Model file for the job. Use its own axes, mm. Coordinates: 2 decimals unless noted, no trailing zeros. Order: outer loops, then holes, each group sorted by start corner. A loop starts at its lowest first (then second) coordinate and runs counter-clockwise, first axis right, second up. Notation, with made-up numbers: M 35.5,-3 L 68.5,-3 A19 ccw 68.5,29 Z; hole C 54,61.5 d3. An arc over 180 degrees is marked long. Return JSON: item names as keys, results as strings.
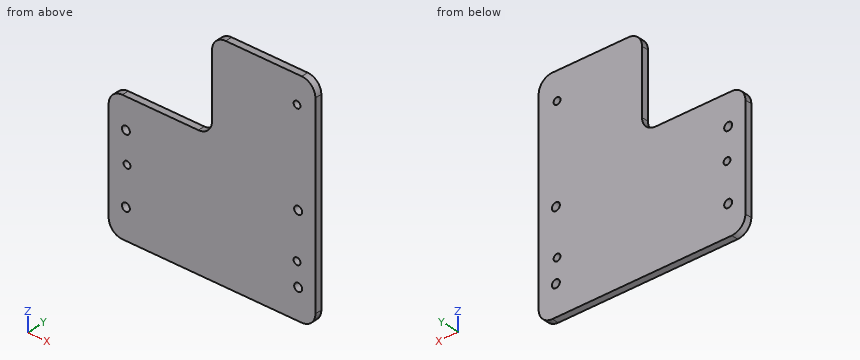
```python
from build123d import *

# Parameters (mm, degrees)
F0_R     = 1.85
F0_R_2   = 1.5875
F1_DEPTH = 3.175


with BuildPart() as f1:
    # F0 (on Front) → F1 (new body)
    with BuildSketch(Plane.XZ):
        with BuildLine():
            ThreePointArc((-48, -23.65), (-46.140128, -28.140128), (-41.65, -30))
            Line((-41.65, -30), (41.65, -30))
            ThreePointArc((41.65, -30), (46.140128, -28.140128), (48, -23.65))
            Line((48, -23.65), (48, 30))
            Line((48, 30), (48, 65.99177))
            ThreePointArc((48, 65.99177), (46.140128, 70.481898), (41.65, 72.34177))
            Line((41.65, 72.34177), (6.35, 72.34177))
            ThreePointArc((6.35, 72.34177), (1.859872, 70.481898), (0, 65.99177))
            Line((0, 65.99177), (0, 36.35))
            ThreePointArc((0, 36.35), (-1.859872, 31.859872), (-6.35, 30))
            Line((-6.35, 30), (-41.65, 30))
            ThreePointArc((-41.65, 30), (-46.140128, 28.140128), (-48, 23.65))
            Line((-48, 23.65), (-48, -23.65))
        make_face()
        with Locations((-40, -16)):
            Circle(F0_R, mode=Mode.SUBTRACT)
        with Locations((-39.4716, 1.8262)):
            Circle(F0_R_2, mode=Mode.SUBTRACT)
        with Locations((-40, 16)):
            Circle(F0_R, mode=Mode.SUBTRACT)
        with Locations((40, -16)):
            Circle(F0_R, mode=Mode.SUBTRACT)
        with Locations((39.4716, -5.362)):
            Circle(F0_R_2, mode=Mode.SUBTRACT)
        with Locations((40, 16)):
            Circle(F0_R, mode=Mode.SUBTRACT)
        with Locations((39.4716, 59.662)):
            Circle(F0_R_2, mode=Mode.SUBTRACT)
    extrude(amount=F1_DEPTH)


solid = f1.part
```
Item 1: Saw through at A-A (z = -16). Write the cut outline in (x, y) (3 decimals), and give its area (3 significant figures).
Check result:
{"outline": "M -48,-3.175 L -41.85,-3.175 L -41.85,0 L -48,0 Z; M -38.15,-3.175 L 38.15,-3.175 L 38.15,0 L -38.15,0 Z; M 41.85,-3.175 L 48,-3.175 L 48,0 L 41.85,0 Z", "area": "281 mm2"}
Item 2: Wall check: line 1 (Z direction, x = 40, y = -1.95); line 2 (Z direction, x = 40.5, y = -1.3); line 3 (X direction, y = -2.7, z = -15.5). Give the ranges that are in metal, low to high.
Check result:
{"line 1": "z = -30 to -17.85, -14.15 to -6.86, -3.87 to 14.15, 17.85 to 58.17, 61.16 to 72.34", "line 2": "z = -30 to -17.78, -14.22 to -6.57, -4.15 to 14.22, 17.78 to 58.45, 60.87 to 72.34", "line 3": "x = -48 to -41.78, -38.22 to 38.22, 41.78 to 48"}
Item 3: Drop flat-ended pins along their axis: pin 1 Ø3.5 at (x, z) = (40, -16) entering from -Y; pin 2 Ø1 at (y, z) = (-1.5, 47) entering from -X; pin 3 Ø1 at (y, z) = (-2, 25.5) entering from -X. Give the stop position or say it passes through.
Check result:
{"pin 1": "passes through", "pin 2": "stops at x = 0", "pin 3": "stops at x = -47.85"}
Item 4: Saw through at C-C (x = -20). Write the cut outline in (y, z) (3 decimals).
Check result:
{"outline": "M -3.175,-30 L 0,-30 L 0,30 L -3.175,30 Z"}
Item 5: Saw through at B-B (y = -1.65). Count the separate pieces of the cut face and the enclosed holes in it, and give its area (3 significant figures).
Check result:
{"separate pieces": "1", "enclosed holes": "7", "area": "7,690 mm2"}
